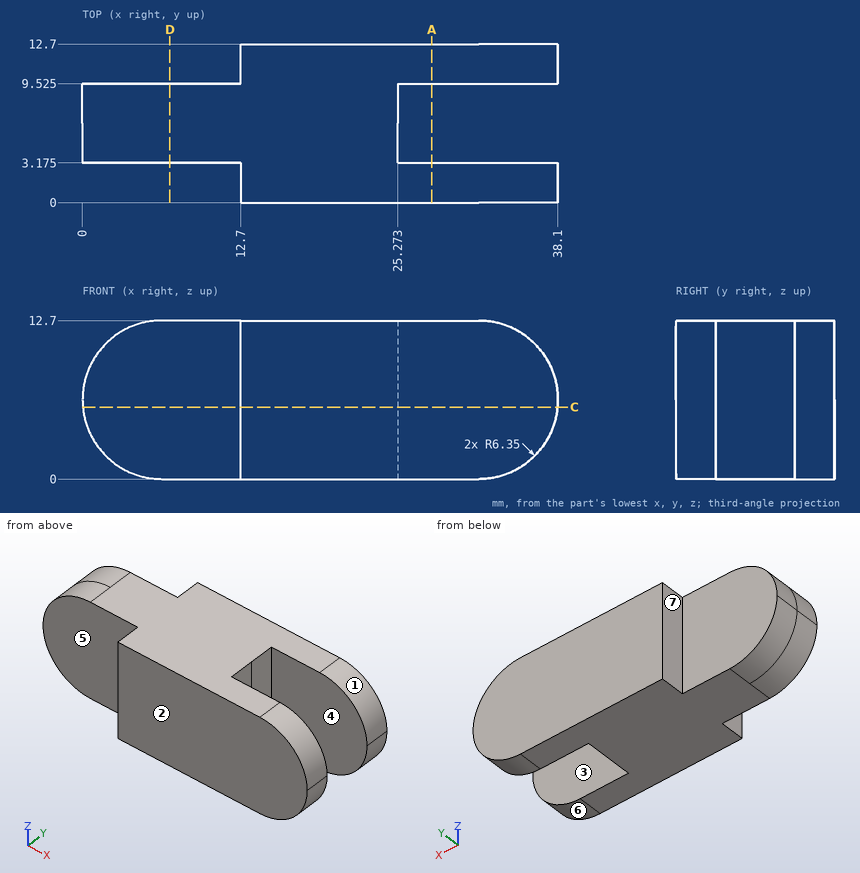
Part print with two shaded views. Sizes in mm from the minimum x, y, z corner. A direction names the side the tool comes from. Coordinates: 2 decimals unless noted, no trailing zeros. Write each loop counter-clockwise with the first axis right and the second up, starting at its lowest first coordinate (ties: lowest second). Pieces come first, ordered by that corner, then holes. Notation, with made-up numbers: (56, 6.25) - (95, 6.25) arc R9 cw to (95, 11.25) - close; hole circle Ø1 at (55.25, 64.25). An arc over 180 degrees is marked (long way). One line per item, written item: value. Start each with the question number.
1. Flat gauge pins, fed straight in: pin 1 (4 mm diameter, centred on x = 7.5, z = 3.5, fed in from -Y) (3 decimals); pin 2 (2.5 mm diameter, centred on y = 5, z = 6.5, fed in from +X); pin 3 (1.6 mm diameter, centred on y = 11.5, z = 9, fed in from -X); pin 4 (6 mm diameter, centred on y = 9, z = 5.5, fed in from +X). Where does each tip first touch, or does it go through?
2. Mould opens along Y. For the marked faces 1, 2 and 3 say: released by +Y, released by -Y, zero draft, split by the parting line, or undercut.
3. Slice it at D-D (x = 7). Write the cut outline in (y, z) (3 decimals), plus the area to 3 significant figures.
4. Tool access for the marked faces 4, 5, 6 and 7: list every direction of +Z, -Z, +X, -X, +Y, -Y with a clear straight run to the whole face (end or side of a thin tool).
5. Slice it at A-A (x = 28). Write the cut outline in (y, z) (3 decimals).
6. Probe line 1 (Y direction, x = 33.5, z = 2) (3 decimals); line 2 (Y direction, x = 6, z = 9.25) (3 decimals); line 3 (X direction, y = 5.5, z = 7.5) (3 decimals). List the from-to ranges inside material, lowest first. Write a range as from..to.
7. Slice it at C-C (z = 5.75). Write the cut outline in (x, y) (3 decimals), plus the area to 3 significant figures.
Answers below:
1. pin 1: stops at y = 3.175
1. pin 2: stops at x = 25.27
1. pin 3: stops at x = 12.7
1. pin 4: stops at x = 38.1
2. face 1: zero draft
2. face 2: released by -Y
2. face 3: undercut
3. outline: (3.175, 0) - (9.525, 0) - (9.525, 12.7) - (3.175, 12.7) - close
3. area: 80.6 mm^2
4. face 4: +Z, -Z, +X
4. face 5: +Z, -Z, -X, -Y
4. face 6: -Z, +X, +Y, -Y
4. face 7: +Z, -Z, -X, +Y
5. outline: (0, 0) - (3.175, 0) - (3.175, 12.7) - (0, 12.7) - close; (9.525, 0) - (12.7, 0) - (12.7, 12.7) - (9.525, 12.7) - close
6. line 1: y = 0..3.175, 9.525..12.7
6. line 2: y = 3.175..9.525
6. line 3: x = 0.105..25.273
7. outline: (0.028, 3.175) - (12.7, 3.175) - (12.7, 0) - (38.072, 0) - (38.072, 3.175) - (25.273, 3.175) - (25.273, 9.525) - (38.072, 9.525) - (38.072, 12.7) - (12.7, 12.7) - (12.7, 9.525) - (0.028, 9.525) - close
7. area: 321 mm^2
